Design review of the part built by this model. Coordinates are the model's own, in mm. Coordinates: 2 decimals unless noted, no trailing zeros. Loops run counter-clockwise (first coordinate to the right, second up) from the corner with the lowest first, then second, coordinate; pieces in that order, holes last. Notation, with made-up numbers: (62, -9.75) -> (81, -9.75) arc R26 cw to (81, 20.25) -> close; hole circle Ø1 at (46, 16). An arc over 180 degrees is marked (long way). One line per item, written item: value. Start each with the question number.
1. Add section A-A on y = 14.5. Write out the cut boundary in (x, z), plus the area to 3 significant figures.
2. For probe 1 along X at (y, z) = (13.75, 1.55); probe 2 along X at (y, z) = (9.5, 0.3); probe 3 along Y at (x, z) = (56.5, 0.55), list the stretches that pass through material, from the lowest coordinate up.
3. Add section B-B on z = 0.95. Give the number of separate pieces and of enclosed holes in the cut face, plus the area to 3 significant figures.
4. Insertion check: pin 1 (0.8 mm diameter, centred on x = 15.5, z = 0.5, fed in from -Y). The pin has a flat end and moves straight along its axis. Give the tip position at first contact, or say it passes through.
```python
from build123d import *

# Parameters (mm, degrees)
SZKIC1_W                    = 91
SZKIC1_H                    = 18
DODANIE_WYCI_GNI_CIE1_DEPTH = 1.6
ZAOKR_GLENIE2_R             = 3.5
SZKIC5_W                    = 2.9
SZKIC5_H                    = 14.52
WYTNIJ_WYCI_GNI_CIE2_DEPTH  = 1.6
SZKIC7_R                    = 1.5
WYTNIJ_WYCI_GNI_CIE3_DEPTH  = 1.6
SZKIC10_R                   = 1.5
WYTNIJ_WYCI_GNI_CIE4_DEPTH  = 1.6
SZKIC11_R                   = 0.75
SZKIC11_R_2                 = 0.750301754
SZKIC11_R_3                 = 0.752070273
SZKIC11_R_4                 = 0.7503443
SZKIC11_R_5                 = 0.750020646
WYTNIJ_WYCI_GNI_CIE5_DEPTH  = 1.6


with BuildPart() as part:
    # Szkic1 → Dodanie-wyciągnięcie1 (new body)
    with BuildSketch(Plane.XY):
        with Locations((14.994318182, 16.981534091)):
            Rectangle(SZKIC1_W, SZKIC1_H)
    extrude(amount=DODANIE_WYCI_GNI_CIE1_DEPTH)

    # Zaokrąglenie2
    zaokr_glenie2_edges = [part.edges().sort_by_distance(p)[0] for p in [
        (60.494318182, 25.981534091, 0.8),
        (60.494318182, 7.981534091, 0.8),
    ]]
    fillet(zaokr_glenie2_edges, radius=ZAOKR_GLENIE2_R)

    # Szkic5 → Wytnij-wyciągnięcie2 (cut)
    with BuildSketch(Plane.XY.offset(1.6)):
        with Locations((-17.255681818, 15.241534091)):
            Rectangle(SZKIC5_W, SZKIC5_H)
        with Locations((-0.755681818, 15.241534091)):
            Rectangle(SZKIC5_W, SZKIC5_H)
        with Locations((15.744318182, 15.241534091)):
            Rectangle(SZKIC5_W, SZKIC5_H)
        with Locations((32.244318182, 15.241534091)):
            Rectangle(SZKIC5_W, SZKIC5_H)
        with Locations((48.744318182, 15.241534091)):
            Rectangle(SZKIC5_W, SZKIC5_H)
    extrude(amount=-WYTNIJ_WYCI_GNI_CIE2_DEPTH, mode=Mode.SUBTRACT)

    # Szkic7 → Wytnij-wyciągnięcie3 (cut)
    with BuildSketch(Plane.XY.offset(1.6)):
        with Locations((-26.305681818, 16.981534091)):
            Circle(SZKIC7_R)
        with Locations((56.294318182, 16.981534091)):
            Circle(SZKIC7_R)
    extrude(amount=-WYTNIJ_WYCI_GNI_CIE3_DEPTH, mode=Mode.SUBTRACT)

    # Szkic10 → Wytnij-wyciągnięcie4 (cut)
    with BuildSketch(Plane.XY.offset(1.6)):
        with Locations((7.494318182, 16.981534091)):
            Circle(SZKIC10_R)
    extrude(amount=-WYTNIJ_WYCI_GNI_CIE4_DEPTH, mode=Mode.SUBTRACT)

    # Szkic11 → Wytnij-wyciągnięcie5 (cut)
    with BuildSketch(Plane(origin=(0, 0, 0), x_dir=(-1, 0, 0), z_dir=(0, 0, -1))):
        with Locations((18.705681818, 21.751534091)):
            Circle(SZKIC11_R)
        with Locations((15.773526009, 21.751534091)):
            Circle(SZKIC11_R)
        with Locations((2.226959067, 21.751534091)):
            Circle(SZKIC11_R_2)
        with Locations((-0.75008283, 21.751534091)):
            Circle(SZKIC11_R_3)
        with Locations((-14.294318182, 21.751534091)):
            Circle(SZKIC11_R)
        with Locations((-17.217046338, 21.751534091)):
            Circle(SZKIC11_R_4)
        with Locations((-30.788753193, 21.751534091)):
            Circle(SZKIC11_R_5)
        with Locations((-33.694318182, 21.751534091)):
            Circle(SZKIC11_R)
        with Locations((-47.294318182, 21.751534091)):
            Circle(SZKIC11_R)
        with Locations((-50.194318182, 21.751534091)):
            Circle(SZKIC11_R)
    extrude(amount=-WYTNIJ_WYCI_GNI_CIE5_DEPTH, mode=Mode.SUBTRACT)


solid = part.part
```
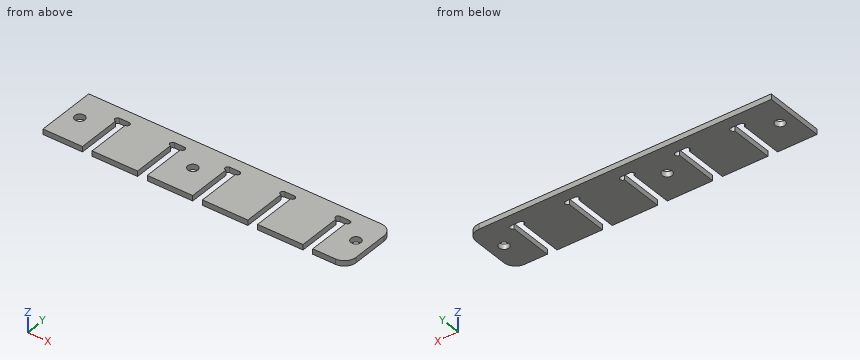
Worked answers:
1. outline: (-30.51, 0) -> (-18.71, 0) -> (-18.71, 1.6) -> (-30.51, 1.6) -> close; (-15.81, 0) -> (-2.21, 0) -> (-2.21, 1.6) -> (-15.81, 1.6) -> close; (0.69, 0) -> (14.29, 0) -> (14.29, 1.6) -> (0.69, 1.6) -> close; (17.19, 0) -> (30.79, 0) -> (30.79, 1.6) -> (17.19, 1.6) -> close; (33.69, 0) -> (47.29, 0) -> (47.29, 1.6) -> (33.69, 1.6) -> close; (50.19, 0) -> (60.49, 0) -> (60.49, 1.6) -> (50.19, 1.6) -> close
1. area: 122 mm²
2. probe 1: x = -30.51 to -18.71, -15.81 to -2.21, 0.69 to 14.29, 17.19 to 30.79, 33.69 to 47.29, 50.19 to 60.49
2. probe 2: x = -30.51 to -18.71, -15.81 to -2.21, 0.69 to 14.29, 17.19 to 30.79, 33.69 to 47.29, 50.19 to 59.88
2. probe 3: y = 7.98 to 15.5, 18.47 to 25.98
3. separate pieces: 1
3. enclosed holes: 3
3. area: 1,390 mm²
4. pin 1: stops at y = 22.5
